from build123d import *


# Not quite as in the source:
# - a feature of the source that left no trace in its solid (it failed there, or was rolled back) is left out


with BuildPart() as f2:
    # F2: sweep along a path in F1
    with BuildLine(Plane.YZ) as f2_path:
        ThreePointArc((0, 0), (269.4076836321, -111.5923163679), (381, -381))
    # F0 (on Front) → F2 (sweep)
    with BuildSketch(Plane.XZ):
        Polygon((76.2, 88.9), (0, 88.9), (-76.2, 88.9), (-76.2, 44.45), (-17.3748321831, 44.45), (-17.3748321831, 0), (-17.3748321831, -44.45), (-76.2, -44.45), (-76.2, -88.9), (0, -88.9), (76.2, -88.9), (76.2, -44.45), (17.3748321831, -44.45), (17.3748321831, 0), (17.3748321831, 44.45), (76.2, 44.45), align=None)
    sweep(path=f2_path.line)


solid = f2.part
Verification items for the finished model (mm, model axes). A direction names the side the tool comes from. Give positions to 0.01 mm unless a question says otherwise; leave off trailing zeros. Loops run counter-clockwise (first coordinate to the right, second up) from the corner with the lowest first, then second, coordinate; pieces in that order, holes last. Notation, with made-up numbers: (60.25, -0.75) - (102.25, -0.75) arc R15 ccw to (102.25, 6.25) - close; hole circle Ø10 at (16.25, -40). An arc over 180 degrees is marked (long way). Write item = value, one per line. Start each with the question number.
Q1. Tool access check on faces 1 (the face through (-46.38, 297.51, -76.87)), 2 (the face through (17.375, 247, -128)), 3 (the face through (76.2, 307, -72)). Record the directions out of +Z, -Z, +X, -X, +Y, -Y that give a thin tool (end or side, any length) a straight path to the whole face; none if there is none.
Q2. Cross-section at D-D, the plane x = -1. Enter the section's corners in (y, z).
Q3. Cross-section at C-C, the plane y = 232. Enter the section's corners in (x, z), and give its area (3 significant figures).
Q4. Depth check by flat-ended pin: P1, Ø12, axis at x = -41.5, z = -139.5, coming from the +Y side; P2, Ø3, axis at x = -57, z = -166.5, coming from the -Y side; P3, Ø10, axis at x = -47, z = -243, coming from the +Y side. Enter the tip coordinate at first touch or a pass-through.
Q5. Mould release check, pull along Y, two halves, no side actions. Record for faces 4 (the face through (1, 0, 1)), 5 (the face through (-76.2, 215, -165)), 6 (the face through (47.2, 297.51, -76.87)): released by +Y, released by -Y, zero draft, split by the parting line, or undercut.
Q6. Thickness scan on line 1 (Y direction, x = -59.5, z = -159); line 2 (Y direction, x = -58.5, z = -313.5); line 3 (Z direction, x = -35.5, y = 267). Record the ranges inside material, lowest first.
Q7. Cross-section at B-B, the plane z = -234.5. Enter the section's corners in (x, y), and give its area (3 significant figures).
Q8. Cross-section at A-A, the plane x = 59.5. Enter the section's corners in (y, z), and give its area (3 significant figures).
Answer key:
q1.face_1 = -X
q1.face_2 = +X
q1.face_3 = +Z, -Z, +X, +Y, -Y
q2.outline = (0, -88.9) arc R292.1 cw to (292.1, -381) - (469.9, -381) arc R469.9 ccw to (0, 88.9) - close
q3.outline = (-76.2, -203.52) - (76.2, -203.52) - (76.2, -137.19) - (17.37, -137.19) - (17.37, -24.37) - (76.2, -24.37) - (76.2, 27.63) - (-76.2, 27.63) - (-76.2, -24.37) - (-17.37, -24.37) - (-17.37, -137.19) - (-76.2, -137.19) - close
q3.area = 22,000 mm^2
q4.P1 = 406.63
q4.P2 = 196.64
q4.P3 = 450.69
q5.face_4 = released by -Y
q5.face_5 = zero draft
q5.face_6 = undercut
q6.line_1 = 189.84 to 252.95, 362.94 to 414.15
q6.line_2 = 284.19 to 329.71, 420.06 to 465.03
q6.line_3 = -262.54 to -176.12, -49.76 to 5.67
q7.outline = (-76.2, 252.71) - (76.2, 252.71) - (76.2, 302.99) - (17.37, 302.99) - (17.37, 399.43) - (76.2, 399.43) - (76.2, 446.48) - (-76.2, 446.48) - (-76.2, 399.43) - (-17.37, 399.43) - (-17.37, 302.99) - (-76.2, 302.99) - close
q7.area = 18,200 mm^2
q8.outline = (0, -88.9) arc R292.1 cw to (292.1, -381) - (336.55, -381) arc R336.55 ccw to (0, -44.45) - close; (0, 44.45) arc R425.45 cw to (425.45, -381) - (469.9, -381) arc R469.9 ccw to (0, 88.9) - close
q8.area = 53,200 mm^2
